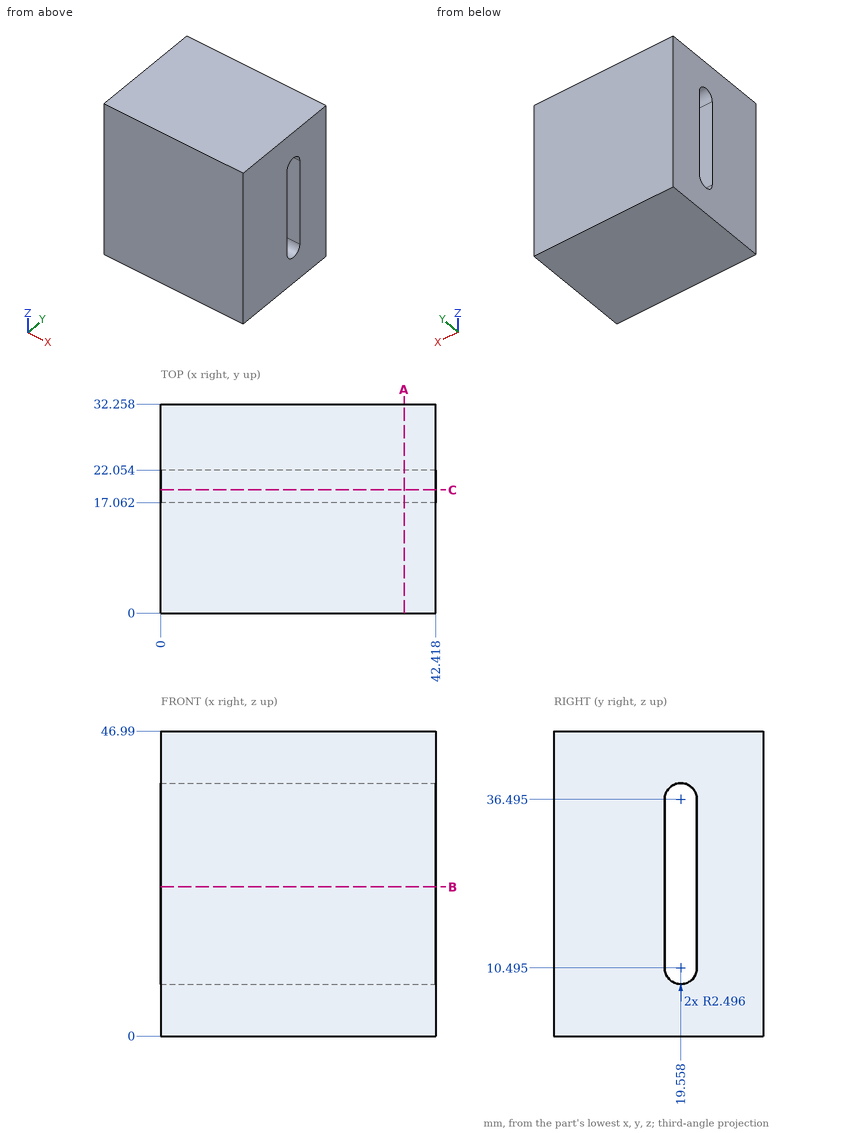
The figure shows three views and two pictorial views of one solid part (mm, origin at its lowest corner). Answer the questions. Round coordinates to 2 decimals unless told otherwise and drop trailing zeros. Order: outer loops, then holes, each group sorted by start corner. A loop starts at its lowest first (then second) coordinate and runs counter-clockwise, first axis right, second up. Notation, with made-up numbers: M 56.25,-15 L 110.25,-15 A13 cw 110.25,3 Z; hole C -32,-32 d3. An arc over 180 degrees is marked long. Put each result on its own line as item: value. Start each with the question number.
Q1. Straight lines are drawn through the part: L1, parallel to Y at x = 34, z = 28.5; L2, parallel to Z at x = 9.5, y = 18 (1 decimal); L3, parallel to Z at x = 8, y = 21. For each, find the intervals that lie inside material, in ascending order. Write a range as [from, to].
Q2. Section A-A, the plane x = 37.5 is taken. Write down the section's boundary in (y, z) (3 decimals), and give its area (3 significant figures).
Q3. Section C-C, the plane y = 19 is taken. Write down the section's boundary in (x, z), and give its area (3 significant figures).
Q4. Section B-B, the plane z = 23 is taken. Write down the section's boundary in (x, y), and give its area (3 significant figures).
Findings below:
1. L1: y = [0, 17.06], [22.05, 32.26]
1. L2: z = [0, 8.5], [38.4, 47]
1. L3: z = [0, 8.46], [38.53, 46.99]
2. outline: M 0,0 L 32.258,0 L 32.258,46.99 L 0,46.99 Z; hole M 17.062,10.495 A2.496 ccw 22.054,10.495 L 22.054,36.495 A2.496 ccw 17.062,36.495 Z
2. area: 1,370 mm^2
3. outline: M 0,0 L 42.42,0 L 42.42,8.06 L 0,8.06 Z; M 0,38.93 L 42.42,38.93 L 42.42,46.99 L 0,46.99 Z
3. area: 684 mm^2
4. outline: M 0,0 L 42.42,0 L 42.42,17.06 L 0,17.06 Z; M 0,22.05 L 42.42,22.05 L 42.42,32.26 L 0,32.26 Z
4. area: 1,160 mm^2
